Design review of the part shown in the three views and the two pictorial views. Dimensions are in mm from the part's minimum x, y and z. Give positions to 0.01 mm unless a question says otherwise; leave off trailing zeros. Loops run counter-clockwise (first coordinate to the right, second up) from the corner with the lowest first, then second, coordinate; pieces in that order, holes last.
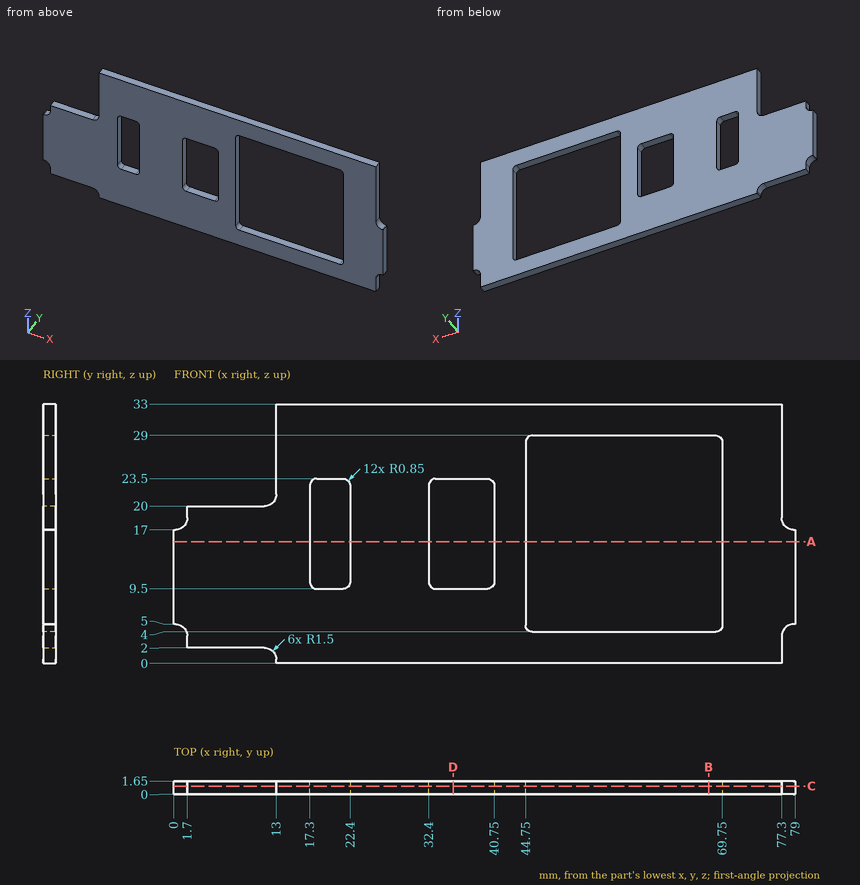
Q1. Consider section B-B on x = 68. Give the boundary of the cut face in (y, z), plus the area to 3 significant figures.
Answers:
outline: (0, 0) - (1.65, 0) - (1.65, 4) - (0, 4) - close; (0, 29) - (1.65, 29) - (1.65, 33) - (0, 33) - close
area: 13.2 mm2
Q2. For pin 1 Ø0.8 at (x, y) = (7.5, 0.5) entering from +Z; pin 2 Ø0.6 at (y, z) = (1, 0) entering from -X; pin 3 Ø0.8 at (y, z) = (0.5, 1) entering from +X, all flat-tipped, find the tip position at first contact; note any pin that passes through.
Answers:
pin 1: stops at z = 20
pin 2: stops at x = 13
pin 3: stops at x = 77.3
Q3. Consider section A-A on z = 15.5. Give the boundary of the cut face in (x, y), plus the area to 3 significant figures.
Answers:
outline: (0, 0) - (17.3, 0) - (17.3, 1.65) - (0, 1.65) - close; (22.4, 0) - (32.4, 0) - (32.4, 1.65) - (22.4, 1.65) - close; (40.75, 0) - (44.75, 0) - (44.75, 1.65) - (40.75, 1.65) - close; (69.75, 0) - (79, 0) - (79, 1.65) - (69.75, 1.65) - close
area: 66.9 mm2
Q4. Consider section D-D on x = 35.5. Give the boundary of the cut face in (y, z).
Answers:
outline: (0, 0) - (1.65, 0) - (1.65, 9.5) - (0, 9.5) - close; (0, 23.5) - (1.65, 23.5) - (1.65, 33) - (0, 33) - close
Q5. Consider section C-C on y = 1.05. Count the separate pieces of the cut face and the enclosed holes in it, plus the area to 3 significant figures.
Answers:
separate pieces: 1
enclosed holes: 3
area: 1,560 mm2
Q6. For probe 1 along X at (y, z) = (1.4, 18.5); probe 2 along X at (y, z) = (1.4, 11); probe 3 along Z at (x, y) = (67, 0.3), list the stretches that pass through material, from the lowest coordinate up.
Answers:
probe 1: x = 1.7 to 17.3, 22.4 to 32.4, 40.75 to 44.75, 69.75 to 77.3
probe 2: x = 0 to 17.3, 22.4 to 32.4, 40.75 to 44.75, 69.75 to 79
probe 3: z = 0 to 4, 29 to 33
